```python
from build123d import *

# Parameters (mm, degrees)
SKETCH010_W     = 70
SKETCH010_H     = 107.5
SKETCH010_R     = 1.5
PAD004_DEPTH    = 4
SKETCH011_R     = 2.5
PAD005_DEPTH    = 5
SKETCH012_R     = 1.5
POCKET001_DEPTH = 4.5


with BuildPart() as part:
    # Sketch010 → Pad004 (new body)
    with BuildSketch(Plane.YZ):
        Rectangle(SKETCH010_W, SKETCH010_H)
        with Locations((-30, 43.75)):
            Circle(SKETCH010_R, mode=Mode.SUBTRACT)
        with Locations((30, 43.75)):
            Circle(SKETCH010_R, mode=Mode.SUBTRACT)
        with Locations((-30, -43.75)):
            Circle(SKETCH010_R, mode=Mode.SUBTRACT)
        with Locations((30, -43.75)):
            Circle(SKETCH010_R, mode=Mode.SUBTRACT)
    extrude(amount=PAD004_DEPTH)

    # Sketch011 (on Face10 of Pad004) → Pad005 (join)
    with BuildSketch(Plane.YZ.offset(4)):
        with Locations((-24.1, 41.25)):
            Circle(SKETCH011_R)
        with Locations((24.1, 39.95)):
            Circle(SKETCH011_R)
        with Locations((-19, -10.85)):
            Circle(SKETCH011_R)
        with Locations((8.9, -10.85)):
            Circle(SKETCH011_R)
        with Locations((24.1, -34.95)):
            Circle(SKETCH011_R)
        with Locations((-24.1, -41.25)):
            Circle(SKETCH011_R)
    extrude(amount=PAD005_DEPTH)

    # Sketch012 (on Face20 of Pad005) → Pocket001 (cut)
    with BuildSketch(Plane.YZ.offset(9)):
        with Locations((-24.1, 41.25)):
            Circle(SKETCH012_R)
        with Locations((24.1, 39.95)):
            Circle(SKETCH012_R)
        with Locations((-19, -10.85)):
            Circle(SKETCH012_R)
        with Locations((8.9, -10.85)):
            Circle(SKETCH012_R)
        with Locations((24.1, -34.95)):
            Circle(SKETCH012_R)
        with Locations((-24.1, -41.25)):
            Circle(SKETCH012_R)
    extrude(amount=-POCKET001_DEPTH, mode=Mode.SUBTRACT)


solid = part.part
```
Build history of the part. All positions in model axes, mm. A direction names the side the tool comes from. Coordinates: 2 decimals unless noted, no trailing zeros. Order: outer loops, then holes, each group sorted by start corner. A loop starts at its lowest first (then second) coordinate and runs counter-clockwise, first axis right, second up. Notation, with made-up numbers: (6, 37.25) -> (55, 37.25) arc R17 cw to (55, 44.25) -> close; hole circle Ø9 at (13, -28.75). An arc over 180 degrees is marked (long way). Answer in a Markdown table with one row per item. Add a question column.
Q1. Drop flat-ended pins along their axis: pin 1 (1.8 mm diameter, centred on y = 30, z = -43.75, fed in from +X); pin 2 (0.9 mm diameter, centred on y = 9, z = -10.5, fed in from +X); pin 3 (4 mm diameter, centred on x = 8, y = 9.5, fed in from +Z). Give the stop position or say it passes through.
Q2. Band-saw the part on A-A, the plane y = 30. List the corners of the cut face in (x, z), then the cut area to 3 significant figures.
Q3. Band-saw the part on D-D, the plane z = -26.5. List the corners of the cut face in (x, y), then the cut area to 3 significant figures.
Q4. Wall check: line 1 along Z through (x, y) = (7.4, -24.1); line 2 along Z through (x, y) = (2.75, -30); line 3 along Z through (x, y) = (5.75, 8.9). Give the ranges that are in metal, low to high. Write a range as [from, to].
Q5. Band-saw the part on C-C, the plane y = -8.5. List the corners of the cut face in (x, z), then the cut area to 3 significant figures.
Q6. Band-saw the part on B-B, the plane z = -10.85. List the corners of the cut face in (x, y), then the cut area to 3 significant figures.
Q7. Mould opens along Y. For faces 3 (the face through (1.972, -30.325, 42.286)), 4 (the face through (9, 26, 40)), 5 (the face through (2, 35, -1)) say: +Y half, -Y half, draft (parallel to the pull), parting line (faces both ways), or undercut.
Q8. Which spindle directions (+Z, -Z, +X, -X, +Y, -Y) get a long thin tool onto all of the face, cutting with end or side? Do faces 1 (the face through (1.97, 28.81, -44.66)), 2 (the face through (6.5, -24.6, 38.8)). Say none if no direction does.
Answers follow:
| question | item | result |
|---|---|---|
| 1 | pin 1 | through |
| 1 | pin 2 | x = 4.5 |
| 1 | pin 3 | z = -8.35 |
| 2 | outline | (0, -53.75) -> (4, -53.75) -> (4, -45.25) -> (0, -45.25) -> close; (0, -42.25) -> (4, -42.25) -> (4, 42.25) -> (0, 42.25) -> close; (0, 45.25) -> (4, 45.25) -> (4, 53.75) -> (0, 53.75) -> close |
| 2 | area | 406 mm^2 |
| 3 | outline | (0, -35) -> (4, -35) -> (4, 35) -> (0, 35) -> close |
| 3 | area | 280 mm^2 |
| 4 | line 1 | [-43.75, -42.75], [-39.75, -38.75], [38.75, 39.75], [42.75, 43.75] |
| 4 | line 2 | [-53.75, -45.25], [-42.25, 42.25], [45.25, 53.75] |
| 4 | line 3 | [-13.35, -12.35], [-9.35, -8.35] |
| 5 | outline | (0, -53.75) -> (4, -53.75) -> (4, 53.75) -> (0, 53.75) -> close |
| 5 | area | 430 mm^2 |
| 6 | outline | (0, -35) -> (4, -35) -> (4, -21.5) -> (9, -21.5) -> (9, -20.5) -> (4.5, -20.5) -> (4.5, -17.5) -> (9, -17.5) -> (9, -16.5) -> (4, -16.5) -> (4, 6.4) -> (9, 6.4) -> (9, 7.4) -> (4.5, 7.4) -> (4.5, 10.4) -> (9, 10.4) -> (9, 11.4) -> (4, 11.4) -> (4, 35) -> (0, 35) -> close |
| 6 | area | 303 mm^2 |
| 7 | face 3 | undercut |
| 7 | face 4 | draft |
| 7 | face 5 | +Y half |
| 8 | face 1 | +X, -X |
| 8 | face 2 | +X |
